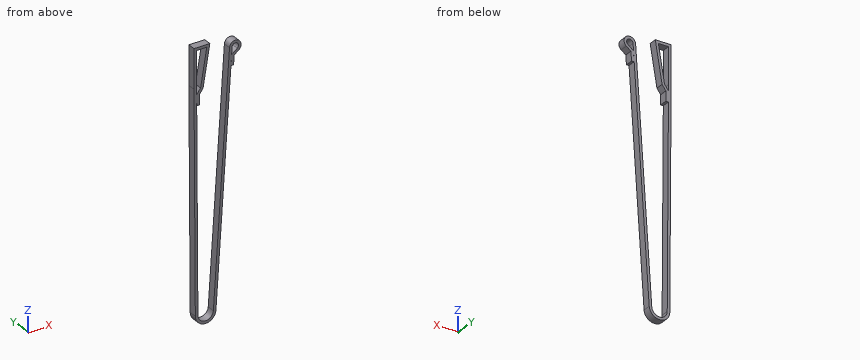
from build123d import *

# Parameters (mm, degrees)
EXTRUDE_THIN3_DEPTH = 3


with BuildPart() as part:
    # Sketch1 → Extrude-Thin3 (new, symmetric)
    with BuildSketch(Plane(origin=(0, 0, 0), x_dir=(1, 0, 0), z_dir=(0, 1, 0))):
        with BuildLine():
            Line((1.127012176, 13.013546351), (1.077715548, 4.681395496))
            Line((1.077715548, 4.681395496), (4.100420922, 0.582923517))
            Line((4.100420922, 0.582923517), (8.897574841, -28.2))
            Line((8.897574841, -28.2), (1, -28.2))
            Line((1, -28.2), (1, -0.002958192))
            Line((1, -0.002958192), (2.00010501, 169.035497988))
            ThreePointArc((2.00010501, 169.035497988), (7.822069743, 174.997361155), (13.987237653, 169.39113333))
            Line((13.987237653, 169.39113333), (26.50957176, -22.293349997))
            ThreePointArc((26.50957176, -22.293349997), (33.11993484, -25.969367239), (33.741089124, -18.431186413))
            Line((33.741089124, -18.431186413), (30.134955883, -15.661433283))
            Line((30.134955883, -15.661433283), (29.667792354, -8.510370309))
            Line((29.667792354, -8.510370309), (27.672046469, -8.640748086))
            Line((27.672046469, -8.640748086), (28.198263672, -16.695769752))
            Line((28.198263672, -16.695769752), (32.522827291, -20.017325785))
            ThreePointArc((32.522827291, -20.017325785), (32.177741578, -24.205204022), (28.505317644, -22.162972221))
            Line((28.505317644, -22.162972221), (15.982983538, 169.521511107))
            ThreePointArc((15.982983538, 169.521511107), (7.762759658, 176.99648154), (0.000140013, 169.04733065))
            Line((0.000140013, 169.04733065), (-1, 0.002958192))
            Line((-1, 0.002958192), (-1, -30.2))
            Line((-1, -30.2), (11.258495684, -30.2))
            Line((11.258495684, -30.2), (5.994431581, 1.384384622))
            Line((5.994431581, 1.384384622), (3.081610843, 5.333864542))
            Line((3.081610843, 5.333864542), (3.126977173, 13.001713688))
            Line((3.126977173, 13.001713688), (1.127012176, 13.013546351))
        make_face()
    extrude(amount=EXTRUDE_THIN3_DEPTH, both=True)


solid = part.part
Source: CAD feature listing. Evaluate the final solid. Frame: model axes, mm. Round coordinates to 2 decimals unless told otherwise and drop trailing zeros. Loops run counter-clockwise (first coordinate to the right, second up) from the corner with the lowest first, then second, coordinate; pieces in that order, holes last. Notation, with made-up numbers: M -18,79.5 L 37,79.5 A14 cw 37,98.5 Z; hole C 69.5,76 d3. An arc over 180 degrees is marked long. Return JSON: item names as keys, results as strings. Group by question number.
1. Section query C-C on z = 2.5. Output: boundary loops of the cut face in (x, y).
2. Section query B-B on y = -0.7. Output: boundary loops of the cut face in (x, z), and give its area (3 significant figures).
3. Material intervals for line 1 along X through (y, z) = (1.3, 22); line 2 along Z through (x, y) = (31, 0.65); line 3 along X through (y, z) = (0, 5), sorted ascending. Write a range as from..to.
4. Pin query (flat end, axial travel): pin 1 (2 mm diameter, centred on y = 0, z = -59.5, fed in from -X); pin 2 (3 mm diameter, centred on y = 0, z = 15.5, fed in from +X); pin 3 (4.5 mm diameter, centred on x = 31, z = 22, fed in from -Y). Return the tip coordinate at first contact, or that it passes through.
5. Section query A-A on z = -137. Output: boundary loops of the cut face in (x, y).
Checks:
{
 "1": {"outline": "M -1,-3 L 1,-3 L 1,3 L -1,3 Z; M 4.61,-3 L 6.64,-3 L 6.64,3 L 4.61,3 Z; M 25.22,-3 L 27.22,-3 L 27.22,3 L 25.22,3 Z"},
 "2": {"outline": "M -1,0 L 0,-169.05 A8 ccw 15.98,-169.52 L 28.51,22.16 A2.5 cw long 32.52,20.02 L 28.2,16.7 L 27.67,8.64 L 29.67,8.51 L 30.13,15.66 L 33.74,18.43 A4.5 ccw long 26.51,22.29 L 13.99,-169.39 A6 cw 2,-169.04 L 1,0 L 1,28.2 L 8.9,28.2 L 4.1,-0.58 L 1.08,-4.68 L 1.13,-13.01 L 3.13,-13 L 3.08,-5.33 L 5.99,-1.38 L 11.26,30.2 L -1,30.2 Z", "area": "984 mm²"},
 "3": {"line 1": "x = -1..1, 7.86..9.89, 26.49..28.49, 33.5..35.5", "line 2": "z = 16.33..18.85, 24.5..26.5", "line 3": "x = -1..1, 5.03..7.06, 25.38..27.38"},
 "4": {"pin 1": "stops at x = -0.65", "pin 2": "stops at x = 31.88", "pin 3": "passes through"},
 "5": {"outline": "M -0.19,-3 L 1.81,-3 L 1.81,3 L -0.19,3 Z; M 16.1,-3 L 18.11,-3 L 18.11,3 L 16.1,3 Z"}
}
